from build123d import *

# Parameters (mm, degrees)
SKETCH1_R           = 38.1
BOSS_EXTRUDE1_DEPTH = 100
SHELL1_T            = -5
SKETCH2_R           = 43.1
SKETCH2_R_2         = 33.1
BOSS_EXTRUDE2_DEPTH = 10
BOSS_EXTRUDE3_DEPTH = 5
CUT_EXTRUDE1_DEPTH  = 5
BOSS_EXTRUDE4_DEPTH = 25.4
CUT_EXTRUDE3_DEPTH  = 50.8
SKETCH9_R           = 3
SKETCH9_W           = 40.386
SKETCH9_H           = 20.32
CUT_EXTRUDE4_DEPTH  = 40.132


with BuildPart() as part:
    # Sketch1 → Boss-Extrude1 (new body)
    with BuildSketch(Plane(origin=(0, 0, 0), x_dir=(1, 0, 0), z_dir=(0, 1, 0))):
        with Locations(Location((0, 0, 0), (0, 0, 270))):
            Circle(SKETCH1_R)
    extrude(amount=BOSS_EXTRUDE1_DEPTH)

    # Shell1
    shell1_openings = [part.faces().sort_by_distance(p)[0] for p in [
        (0, 100, 0),
        (0, 0, 0),
    ]]
    offset(amount=SHELL1_T, openings=shell1_openings, kind=Kind.INTERSECTION)

    # Sketch2 → Boss-Extrude2 (add)
    with BuildSketch(Plane.XZ):
        with Locations(Location((0, 0, 0), (0, 0, 270))):
            Circle(SKETCH2_R)
        with Locations(Location((0, 0, 0), (0, 0, 270))):
            Circle(SKETCH2_R_2, mode=Mode.SUBTRACT)
    extrude(amount=BOSS_EXTRUDE2_DEPTH)

    # Sketch4 → Boss-Extrude3 (add)
    with BuildSketch(Plane.XZ.offset(10)):
        with BuildLine():
            ThreePointArc((-13, 30.440269381), (-5.381039934, 0), (-13, -30.440269381))
            ThreePointArc((-13, -30.440269381), (0, -33.1), (13, -30.440269381))
            ThreePointArc((13, -30.440269381), (5.381039934, 0), (13, 30.440269381))
            ThreePointArc((13, 30.440269381), (0, 33.1), (-13, 30.440269381))
        make_face()
    extrude(amount=-BOSS_EXTRUDE3_DEPTH)

    # Sketch5 → Cut-Extrude1 (cut)
    with BuildSketch(Plane.XZ.offset(10)):
        with BuildLine():
            Line((-2, 1.5), (2, 1.5))
            ThreePointArc((2, 1.5), (2.5, 0), (2, -1.5))
            Line((2, -1.5), (-2, -1.5))
            ThreePointArc((-2, -1.5), (-2.5, 0), (-2, 1.5))
        make_face()
    extrude(amount=-CUT_EXTRUDE1_DEPTH, mode=Mode.SUBTRACT)

    # Sketch6 → Boss-Extrude4 (add)
    with BuildSketch(Plane(origin=(0, 100, 0), x_dir=(1, 0, 0), z_dir=(0, 1, 0))):
        with BuildLine():
            Line((18, 33.579904705), (18, -33.579904705))
            ThreePointArc((18, -33.579904705), (-38.1, 0), (18, 33.579904705))
        make_face()
    extrude(amount=-BOSS_EXTRUDE4_DEPTH)

    # Sketch8 → Cut-Extrude3 (cut)
    with BuildSketch(Plane(origin=(0, 100, 0), x_dir=(1, 0, 0), z_dir=(0, 1, 0))):
        with BuildLine():
            Line((18, -42.955320998), (18, 42.955320998))
            ThreePointArc((18, 42.955320998), (52.271949939, 0), (18, -42.955320998))
        make_face()
    extrude(amount=-CUT_EXTRUDE3_DEPTH, mode=Mode.SUBTRACT)

    # Sketch9 → Cut-Extrude4 (cut)
    with BuildSketch(Plane(origin=(18, 0, 0), x_dir=(0, 0, -1), z_dir=(1, 0, 0))):
        with Locations((-24.13, 94.666)):
            Circle(SKETCH9_R)
        with Locations((-24.13, 85.014)):
            Circle(SKETCH9_R)
        with Locations(Location((24.13, 85.014, 0), (0, 0, 180))):
            Circle(SKETCH9_R)
        with Locations(Location((24.13, 94.666, 0), (0, 0, 180))):
            Circle(SKETCH9_R)
        with Locations((0, 89.84)):
            Rectangle(SKETCH9_W, SKETCH9_H)
    extrude(amount=-CUT_EXTRUDE4_DEPTH, mode=Mode.SUBTRACT)


solid = part.part
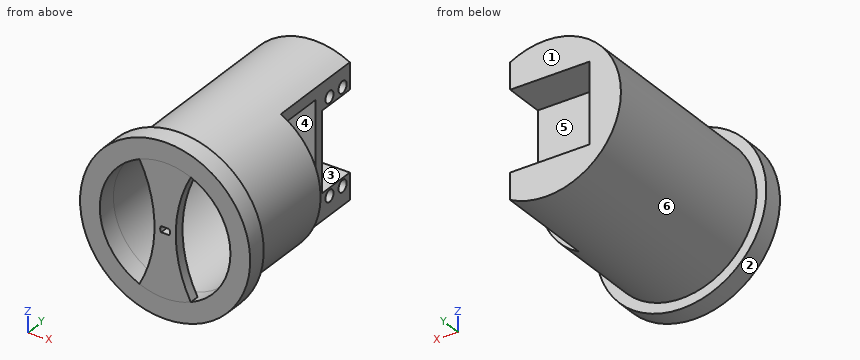
Work out the finished part from the listing and answer in its coordinate system (mm). Face numbers are marked on the shaded views. A direction names the side the tool comes from. Coordinates: 2 decimals unless noted, no trailing zeros. Write each loop counter-clockwise with the first axis right and the second up, starting at its lowest first coordinate (ties: lowest second). Pieces come first, ordered by that corner, then holes.
1. For the marked faces 4, 5 and 6, determine the directions among +Z, -Z, +X, -X, +Y, -Y from which every point of the face is accessible in a straight line to the end or side of a thin tool.
Results list:
face 4: none
face 5: +X, +Y
face 6: +Y
2. The part is cut by section C-C, the plane x = 0. Write down the section's boundary in (y, z), and give its area (3 significant figures).
Results list:
outline: (-10, -43.1) - (0, -43.1) - (0, -38.1) - (100, -38.1) - (100, -20.19) - (79.68, -20.19) - (79.68, 20.19) - (100, 20.19) - (100, 38.1) - (0, 38.1) - (0, 43.1) - (-10, 43.1) - (-10, 1.5) - (-5, 1.5) - (-5, 33.1) - (74.6, 33.1) - (74.6, -33.1) - (-5, -33.1) - (-5, -1.5) - (-10, -1.5) - close; hole circle Ø6 at (85.01, -24.13); hole circle Ø6 at (85.01, 24.13); hole circle Ø6 at (94.67, -24.13); hole circle Ø6 at (94.67, 24.13)
area: 2,260 mm2
3. The part is cut by section B-B, the plane x = 23. Write down the section's boundary in (y, z), and give its area (3 significant figures).
Results list:
outline: (-10, -36.45) - (0, -36.45) - (0, -30.37) - (49.2, -30.37) - (49.2, -23.8) - (-10, -23.8) - close; (-10, 23.8) - (49.2, 23.8) - (49.2, 30.37) - (0, 30.37) - (0, 36.45) - (-10, 36.45) - close
area: 900 mm2
4. Consider line 1 along Y through (x, z) = (-12.5, 24.13); line 2 along Y through (x, z) = (-11, -24.5); line 3 along Y through (x, z) = (6, -24). Determine where each line is inside the solid, lowest interval first.
Results list:
line 1: y = 74.6 to 82.01, 88.01 to 91.67, 97.67 to 100
line 2: y = 74.6 to 82.04, 87.99 to 91.69, 97.64 to 100
line 3: y = -10 to -5, 74.6 to 82.02, 88.01 to 91.67, 97.66 to 100
5. The part is cut by section D-D, the plane y = 40. Write down the section's boundary in (x, z).
Results list:
outline: circle Ø76.2 at (0, 0); hole circle Ø66.2 at (0, 0)
6. The part is cut by section A-A, the plane z = 5. Write down the section's boundary in (x, y), and give its area (3 significant figures).
Results list:
outline: (-42.81, -10) - (-32.72, -10) - (-32.72, 74.6) - (18, 74.6) - (18, 79.68) - (-22.13, 79.68) - (-22.13, 100) - (-37.77, 100) - (-37.77, 0) - (-42.81, 0) - close; (-5.57, -10) - (5.57, -10) - (5.57, -5) - (-5.57, -5) - close; (32.72, -10) - (42.81, -10) - (42.81, 0) - (37.77, 0) - (37.77, 49.2) - (32.72, 49.2) - close
area: 1,480 mm2
7. Flat-ended cylindrical pins translate along their axes: pin 1 (12 mm diameter, centred on y = 1.5, z = -29, fed in from -X); pin 2 (15.5 mm diameter, centred on x = -14.5, z = -9.5, fed in from -Y); pin 3 (1 mm diameter, centred on y = 57.5, z = 3, fed in from -X). Find the tip coordinate at first contact, or state that the pin passes through.
Results list:
pin 1: stops at x = -36.33
pin 2: stops at y = 74.6
pin 3: stops at x = -38.02
8. For a pull along Z with two mould halves and no side action, classify the marked faces 1, 2 and 3 as +Z half, -Z half, draft (parallel to the pull), parting line (faces both ways), or undercut.
Results list:
face 1: draft
face 2: parting line
face 3: undercut
